CAD build for the part. Positions are in the model's coordinates, mm. Face numbers are marked on the shaded views. Round coordinates to 2 decimals unless told otherwise and drop trailing zeros. Order: outer loops, then holes, each group sorted by start corner. A loop starts at its lowest first (then second) coordinate and runs counter-clockwise, first axis right, second up. Notation, with made-up numbers: (-33, 45) - (19, 45) arc R29 ccw to (19, 78) - close; hole circle Ø8 at (81.5, -29.75). An arc over 180 degrees is marked (long way). Use one line per item in the form item = value. Start each with the question number.
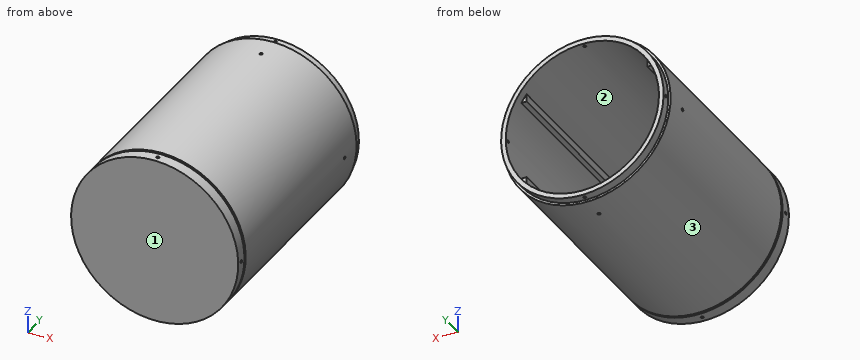
from build123d import *

# Parameters (mm, degrees)
SKETCH_6_R               = 72
SKETCH_6_R_2             = 70
EXTRUDE_1_DEPTH          = 190
SKETCH_6_15_R            = 70
SKETCH_6_15_R_2          = 66
EXTRUDE_2_DEPTH          = 197.5
SKETCH_6_16_R            = 66
EXTRUDE_3_DEPTH          = 3
EXTRUDE_6_DEPTH          = 190
F_2_5MM_3_D              = 2.5
F_2_5MM_3_DEPTH          = 70
PATTERN_CIRCULAR_1_COUNT = 4
SKETCH_33_W              = 1
SKETCH_33_H              = 2
PATTERN_CIRCULAR_2_COUNT = 4
PATTERN_CIRCULAR_3_COUNT = 4


with BuildPart() as part:
    # 草圖6 → 填料-伸長1 (new body)
    with BuildSketch(Plane(origin=(0, 0, 0), x_dir=(1, 0, 0), z_dir=(0, 1, 0))):
        with Locations(Location((0, 0, 0), (0, 0, 270))):
            Circle(SKETCH_6_R)
        with Locations(Location((0, 0, 0), (0, 0, 270))):
            Circle(SKETCH_6_R_2, mode=Mode.SUBTRACT)
    extrude(amount=EXTRUDE_1_DEPTH)

    # 草圖6<15> → 填料-伸長2 (add)
    with BuildSketch(Plane(origin=(0, 0, 0), x_dir=(1, 0, 0), z_dir=(0, 1, 0))):
        with Locations(Location((0, 0, 0), (0, 0, 90))):
            Circle(SKETCH_6_15_R)
        with Locations(Location((0, 0, 0), (0, 0, 90))):
            Circle(SKETCH_6_15_R_2, mode=Mode.SUBTRACT)
    extrude(amount=EXTRUDE_2_DEPTH)

    # 草圖6<16> → 填料-伸長3 (add)
    with BuildSketch(Plane(origin=(0, 0, 0), x_dir=(1, 0, 0), z_dir=(0, 1, 0))):
        with Locations(Location((0, 0, 0), (0, 0, 90))):
            Circle(SKETCH_6_16_R)
    extrude(amount=EXTRUDE_3_DEPTH)

    # 草圖9 → 填料-伸長6 (add)
    with BuildSketch(Plane(origin=(0, 0, 0), x_dir=(1, 0, 0), z_dir=(0, 1, 0))):
        with BuildLine():
            Line((-52, 34), (-52, 40.644802866))
            ThreePointArc((-52, 40.644802866), (-54.38584794, 37.392239086), (-56.568542495, 34))
            Line((-56.568542495, 34), (-52, 34))
        make_face()
        with BuildLine():
            Line((-52, -34), (-56.568542495, -34))
            ThreePointArc((-56.568542495, -34), (-54.38584794, -37.392239086), (-52, -40.644802866))
            Line((-52, -40.644802866), (-52, -34))
        make_face()
        with BuildLine():
            Line((56.568542495, -34), (52, -34))
            Line((52, -34), (52, -40.644802866))
            ThreePointArc((52, -40.644802866), (54.38584794, -37.392239086), (56.568542495, -34))
        make_face()
        with BuildLine():
            ThreePointArc((56.568542495, 34), (54.38584794, 37.392239086), (52, 40.644802866))
            Line((52, 40.644802866), (52, 34))
            Line((52, 34), (56.568542495, 34))
        make_face()
    extrude(amount=EXTRUDE_6_DEPTH)

    # Ø2.5mm 定位孔3
    with Locations(Plane(origin=(70, 193.75, 0), x_dir=(0, 0, 1), z_dir=(1, 0, 0))):
        with Locations((0, 0)):
            f_2_5mm_3 = Hole(F_2_5MM_3_D / 2, depth=F_2_5MM_3_DEPTH)

    # 環狀複製排列1: Ø2.5mm 定位孔3 ×4 about axis
    pattern_circular_1_axis = Axis((0, 197.5, 0), (0, 1, 0))
    for i in range(1, PATTERN_CIRCULAR_1_COUNT):
        add(f_2_5mm_3.rotate(pattern_circular_1_axis, i * 360 / PATTERN_CIRCULAR_1_COUNT), mode=Mode.SUBTRACT)

    # 草圖33 → 除料-旋轉1 (revolve, cut)
    with BuildSketch(Plane.XY, mode=Mode.PRIVATE) as cut_revolve_1_sk:
        with Locations((-71.5, 11)):
            Rectangle(SKETCH_33_W, SKETCH_33_H)
    revolve(cut_revolve_1_sk.sketch.rotate(Axis((0, 197.5, 0), (0, -1, 0)), 270), axis=Axis((0, 197.5, 0), (0, -1, 0)), mode=Mode.SUBTRACT)

    # 草圖37 → Ø2.5mm 定位孔4 (revolve, cut)
    with BuildSketch(Plane(origin=(-72, 5, 0), x_dir=(0, 0, 1), z_dir=(0, 1, 0))):
        Polygon((0, 0), (0, 4.751075774), (1.25, 4), (1.25, 0), align=None)
    f_2_5mm_4 = revolve(axis=Axis((-78.35, 5, 0), (1, 0, 0)), mode=Mode.SUBTRACT)

    # 環狀複製排列2: Ø2.5mm 定位孔4 ×4 about axis
    pattern_circular_2_axis = Axis((0, 197.5, 0), (0, -1, 0))
    for i in range(1, PATTERN_CIRCULAR_2_COUNT):
        add(f_2_5mm_4.rotate(pattern_circular_2_axis, i * 360 / PATTERN_CIRCULAR_2_COUNT), mode=Mode.SUBTRACT)

    # 草圖38 → Ø2.5mm 定位孔5 (revolve, cut)
    with BuildSketch(Plane(origin=(-72, 170.901826282, 0), x_dir=(0, 0, 1), z_dir=(0, 1, 0))):
        Polygon((0, 0), (0, 4.751075774), (1.25, 4), (1.25, 0), align=None)
    f_2_5mm_5 = revolve(axis=Axis((-78.35, 170.901826282, 0), (1, 0, 0)), mode=Mode.SUBTRACT)

    # 環狀複製排列3: Ø2.5mm 定位孔5 ×4 about axis
    pattern_circular_3_axis = Axis((0, 197.5, 0), (0, -1, 0))
    for i in range(1, PATTERN_CIRCULAR_3_COUNT):
        add(f_2_5mm_5.rotate(pattern_circular_3_axis, i * 360 / PATTERN_CIRCULAR_3_COUNT), mode=Mode.SUBTRACT)


solid = part.part
(1) Mould opens along Z. For the marked faces 1, 2 and 3 say: pulls with the +Z half, pulls with the -Z half, needs draft (parallel to the pull), parting line crosses it, or undercut.
(2) Slice it at A-A (y = 176). Give the cut face in (x, z), and give its area (3 significant figures).
(3) Slice it at B-B (x = -7.5). Give the cut face in (y, z), and give its area (3 significant figures).
(4) Flat gauge pins, fed straight in: P1, Ø1, axis at y = 165.5, z = -15.5, coming from the -X side; P2, Ø3.5, axis at y = 50.5, z = -36, coming from the -X side; P3, Ø4, axis at x = 0, y = 170.9, coming from the +Z side; P4, Ø7.5, axis at y = 63, z = 36, coming from the -X side. Where does each tip first touch, or does it go through?
(5) Wall check: line 1 (Y direction, x = 70.05, z = 0); line 2 (Y direction, x = 71.2, z = 0); line 3 (Y direction, x = -69, z = 0). Give the ranges that are in metal, low to high. Write a range as [from, to].
(6) Slice it at C-C (z = 4). Give the cut face in (x, y), and give its area (3 significant figures).
Results list:
q1.face_1 = needs draft
q1.face_2 = undercut
q1.face_3 = parting line crosses it
q2.outline = circle Ø144 at (0, 0); hole (-56.57, -34) - (-52, -34) - (-52, -40.64) arc R66 ccw to (52, -40.64) - (52, -34) - (56.57, -34) arc R66 ccw to (56.57, 34) - (52, 34) - (52, 40.64) arc R66 ccw to (-52, 40.64) - (-52, 34) - (-56.57, 34) arc R66 ccw to start
q2.area = 2,660 mm²
q3.outline = (0, -71.61) - (10, -71.61) - (10, -70.6) - (12, -70.6) - (12, -71.61) - (190, -71.61) - (190, -69.6) - (197.5, -69.6) - (197.5, -65.57) - (3, -65.57) - (3, 65.57) - (197.5, 65.57) - (197.5, 69.6) - (190, 69.6) - (190, 71.61) - (12, 71.61) - (12, 70.6) - (10, 70.6) - (10, 71.61) - (0, 71.61) - close
q3.area = 2,740 mm²
q4.P1 = -70.42
q4.P2 = -63.33
q4.P3 = 72
q4.P4 = -64.37
q5.line_1 = [0, 3.75], [6.25, 169.65], [172.15, 190]
q5.line_2 = [0, 3.75], [6.25, 10], [12, 169.65], [172.15, 190]
q5.line_3 = [0, 3.75], [6.25, 169.65], [172.15, 192.5], [195, 197.5]
q6.outline = (-71.89, 0) - (71.89, 0) - (71.89, 10) - (70.89, 10) - (70.89, 12) - (71.89, 12) - (71.89, 190) - (69.89, 190) - (69.89, 197.5) - (65.88, 197.5) - (65.88, 3) - (-65.88, 3) - (-65.88, 197.5) - (-69.89, 197.5) - (-69.89, 190) - (-71.89, 190) - (-71.89, 12) - (-70.89, 12) - (-70.89, 10) - (-71.89, 10) - close
q6.area = 2,740 mm²
